Design review of the part built by this model. Coordinates are the model's own, in mm. Give positions to 0.01 mm unless a question says otherwise; leave off trailing zeros. Loops run counter-clockwise (first coordinate to the right, second up) from the corner with the lowest first, then second, coordinate; pieces in that order, holes last. Notation, with made-up numbers: (-13, -5.5) -> (22, -5.5) arc R35 cw to (22, 27.5) -> close; hole circle Ø10 at (84, -1). An arc over 180 degrees is marked (long way). Answer in a Markdown table with one row per item. Add a question column.
(1) For pin 1 (2 mm diameter, centred on x = -177.5, z = -88.5, fed in from -Y); pin 2 (1.6 mm diameter, centred on x = -135, y = -1.5, fed in from +Z), all flat-tipped, find the tip position at first contact; note any pin that passes through.
(2) Consider section B-B on x = -262. Write out the cut boundary in (y, z) (3 decimals), then the cut area to 3 significant figures.
(3) Consider section A-A on z = 46. Count the separate pieces of the cut face and the enclosed holes in it, then the cut area to 3 significant figures.
(4) For line 1 (Z direction, x = -31, y = -0.6); line 2 (Z direction, x = -201.5, y = -1), list the stretches that pass through material, from the lowest coordinate up.
from build123d import *

# Parameters (mm, degrees)
F0_W     = 609.6
F0_H     = 304.8
F1_DEPTH = 3.175
F2_W     = 45.72
F2_H     = 3.175
F2_W_2   = 28.575
F3_DEPTH = 254
F4_R     = 5.08
F5_R     = 5.08


with BuildPart() as f1:
    # F0 (on Front) → F1 (new body)
    with BuildSketch(Plane.XZ):
        Rectangle(F0_W, F0_H)
    extrude(amount=F1_DEPTH)

    # F2 (on face) → F3 (cut)
    with BuildSketch(Plane.XY.offset(152.4)):
        with Locations((-251.46, -1.5875)):
            Rectangle(F2_W, F2_H)
        with Locations((-188.9125, -1.5875)):
            Rectangle(F2_W_2, F2_H)
        with Locations((-134.9375, -1.5875)):
            Rectangle(F2_W_2, F2_H)
        with Locations((-80.9625, -1.5875)):
            Rectangle(F2_W_2, F2_H)
        with Locations((-26.9875, -1.5875)):
            Rectangle(F2_W_2, F2_H)
        with Locations((26.9875, -1.5875)):
            Rectangle(F2_W_2, F2_H)
        with Locations((80.9625, -1.5875)):
            Rectangle(F2_W_2, F2_H)
        with Locations((134.9375, -1.5875)):
            Rectangle(F2_W_2, F2_H)
        with Locations((188.9125, -1.5875)):
            Rectangle(F2_W_2, F2_H)
        with Locations((251.46, -1.5875)):
            Rectangle(F2_W, F2_H)
    extrude(amount=-F3_DEPTH, mode=Mode.SUBTRACT)

    # F4
    f4_edges = [f1.edges().sort_by_distance(p)[0] for p in [
        (-274.32, -1.5875, 152.4),
        (-228.6, -1.5875, 152.4),
        (-228.6, -1.5875, -101.6),
        (-274.32, -1.5875, -101.6),
        (-304.8, -1.5875, 152.4),
        (304.8, -1.5875, 152.4),
        (-203.2, -1.5875, 152.4),
        (-174.625, -1.5875, 152.4),
        (-149.225, -1.5875, 152.4),
        (-120.65, -1.5875, 152.4),
        (-95.25, -1.5875, 152.4),
        (-66.675, -1.5875, 152.4),
        (-41.275, -1.5875, 152.4),
        (-12.7, -1.5875, 152.4),
        (12.7, -1.5875, 152.4),
        (66.675, -1.5875, 152.4),
        (95.25, -1.5875, 152.4),
        (149.225, -1.5875, 152.4),
        (41.275, -1.5875, 152.4),
        (120.65, -1.5875, 152.4),
        (174.625, -1.5875, 152.4),
        (228.6, -1.5875, 152.4),
        (274.32, -1.5875, 152.4),
        (203.2, -1.5875, 152.4),
    ]]
    fillet(f4_edges, radius=F4_R)

    # F5
    f5_edges = [f1.edges().sort_by_distance(p)[0] for p in [
        (-174.625, -1.5875, -101.6),
        (-120.65, -1.5875, -101.6),
        (-66.675, -1.5875, -101.6),
        (-12.7, -1.5875, -101.6),
        (41.275, -1.5875, -101.6),
        (95.25, -1.5875, -101.6),
        (149.225, -1.5875, -101.6),
        (203.2, -1.5875, -101.6),
        (274.32, -1.5875, -101.6),
        (228.6, -1.5875, -101.6),
        (174.625, -1.5875, -101.6),
        (120.65, -1.5875, -101.6),
        (66.675, -1.5875, -101.6),
        (12.7, -1.5875, -101.6),
        (-41.275, -1.5875, -101.6),
        (-95.25, -1.5875, -101.6),
        (-149.225, -1.5875, -101.6),
        (-203.2, -1.5875, -101.6),
    ]]
    fillet(f5_edges, radius=F5_R)


solid = f1.part
Values follow:
| question | item | result |
|---|---|---|
| 1 | pin 1 | through |
| 1 | pin 2 | z = -101.6 |
| 2 | outline | (-3.175, -152.4) -> (0, -152.4) -> (0, -101.6) -> (-3.175, -101.6) -> close |
| 2 | area | 161 mm2 |
| 3 | separate pieces | 11 |
| 3 | enclosed holes | 0 |
| 3 | area | 919 mm2 |
| 4 | line 1 | -152.4 to -101.6 |
| 4 | line 2 | -152.4 to -100.31 |
